```python
from build123d import *

# Parameters (mm, degrees)
SKETCH1_W      = 400
SKETCH1_H      = 500
EXTRUDE1_DEPTH = 10
SHELL1_T       = -5


with BuildPart() as part:
    # Sketch1 → Extrude1 (new body)
    with BuildSketch(Plane(origin=(0, 0, 0), x_dir=(1, 0, 0), z_dir=(0, 1, 0))):
        with Locations((200, 250)):
            Rectangle(SKETCH1_W, SKETCH1_H)
    extrude(amount=-EXTRUDE1_DEPTH)

    # Shell1
    shell1_openings = [part.faces().sort_by_distance(p)[0] for p in [
        (200, 0, -250),
    ]]
    offset(amount=SHELL1_T, openings=shell1_openings, kind=Kind.INTERSECTION)


solid = part.part
```
Build history of the part. All positions in model axes, mm. Round coordinates to 2 decimals unless told otherwise and drop trailing zeros. Loops run counter-clockwise (first coordinate to the right, second up) from the corner with the lowest first, then second, coordinate; pieces in that order, holes last.
Item 1: Drill centre lines: line 1 along X through (y, z) = (-4.5, -156); line 2 along Z through (x, y) = (168, -1.5); line 3 along Y through (x, z) = (369, -443.5). Where is each one in solid material? Low to high.
Item 2: Saw through at B-B (z = -375). List the corners of the cut face in (x, y), then the cut area to 3 significant figures.
Item 3: Saw through at C-C (x = 53). List the corners of the cut face in (y, z), then the cut area to 3 significant figures.
Item 4: Saw through at A-A (y = -1.5). List the corners of the cut face in (x, z), then the cut area to 3 significant figures.
Item 5: Pin check, flat tips, straight feed: P1, Ø4, axis at x = 206.5, y = -4.5, coming from the +Z side; P2, Ø3, axis at x = 340, z = -367, coming from the +Y side. Stop position of each tip, or through.
Item 6: Two-plate mould, pull along Z, no slides. Class faces 1 (the face through (197, -10, -254)), 2 (the face through (197, -5, -253)), 3 (the face through (197, -5, 0)), 4 (the face through (197, -5, -500)): released by +Z, released by -Z, zero draft, split by the parting line, or undercut.
Worked answers:
1. line 1: x = 0 to 5, 395 to 400
1. line 2: z = -500 to -495, -5 to 0
1. line 3: y = -10 to -5
2. outline: (0, -10) - (400, -10) - (400, 0) - (395, 0) - (395, -5) - (5, -5) - (5, 0) - (0, 0) - close
2. area: 2,050 mm2
3. outline: (-10, -500) - (0, -500) - (0, -495) - (-5, -495) - (-5, -5) - (0, -5) - (0, 0) - (-10, 0) - close
3. area: 2,550 mm2
4. outline: (0, -500) - (400, -500) - (400, 0) - (0, 0) - close; hole (5, -495) - (395, -495) - (395, -5) - (5, -5) - close
4. area: 8,900 mm2
5. P1: stops at z = 0
5. P2: stops at y = -5
6. face 1: zero draft
6. face 2: undercut
6. face 3: released by +Z
6. face 4: released by -Z
